For this review, take the finished solid that the model builds, in its own axes (mm). Give positions to 0.01 mm unless a question says otherwise; leave off trailing zeros. Write each loop counter-clockwise with the first axis right and the second up, starting at its lowest first coordinate (ties: lowest second). Pieces come first, ordered by that corner, then holes. Notation, with made-up numbers: M 2,74 L 59,74 A20 ccw 59,97 Z; hole C 51,24 d1. An arc over 180 degrees is marked long. Write item = value, one per line.
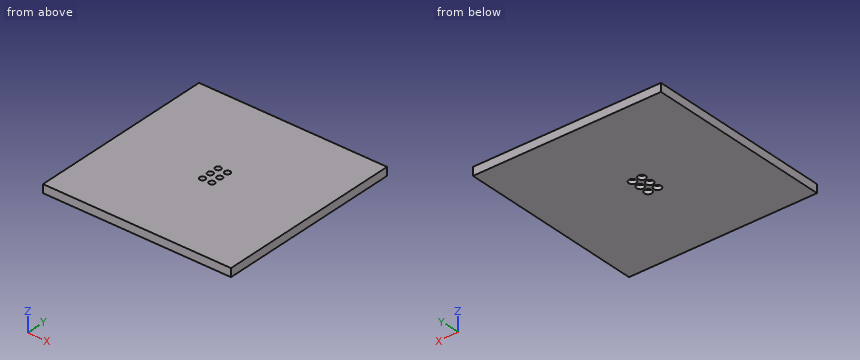
```python
from build123d import *

# Parameters (mm, degrees)
F0_W     = 50
F0_H     = 50
F0_R     = 0.75
F1_DEPTH = 1.2
F2_W     = 50
F2_H     = 50
F2_R     = 1
F3_DEPTH = 1


with BuildPart() as f1:
    # F0 (on Top) → F1 (new body)
    with BuildSketch(Plane.XY):
        Rectangle(F0_W, F0_H)
        with Locations((-1.25, -2.5)):
            Circle(F0_R, mode=Mode.SUBTRACT)
        with Locations((1.25, -2.5)):
            Circle(F0_R, mode=Mode.SUBTRACT)
        with Locations((-1.25, 0)):
            Circle(F0_R, mode=Mode.SUBTRACT)
        with Locations((-1.25, 2.5)):
            Circle(F0_R, mode=Mode.SUBTRACT)
        with Locations((1.25, 0)):
            Circle(F0_R, mode=Mode.SUBTRACT)
        with Locations((1.25, 2.5)):
            Circle(F0_R, mode=Mode.SUBTRACT)
    extrude(amount=F1_DEPTH)

    # F2 (on face) → F3 (join)
    with BuildSketch(Plane(origin=(0, 0, 0), x_dir=(1, 0, 0), z_dir=(0, 0, -1))):
        Rectangle(F2_W, F2_H)
        with Locations((-1.25, -2.5)):
            Circle(F2_R, mode=Mode.SUBTRACT)
        with Locations((1.25, -2.5)):
            Circle(F2_R, mode=Mode.SUBTRACT)
        with Locations((-1.25, 0)):
            Circle(F2_R, mode=Mode.SUBTRACT)
        with Locations((-1.25, 2.5)):
            Circle(F2_R, mode=Mode.SUBTRACT)
        with Locations((1.25, 0)):
            Circle(F2_R, mode=Mode.SUBTRACT)
        with Locations((1.25, 2.5)):
            Circle(F2_R, mode=Mode.SUBTRACT)
    extrude(amount=F3_DEPTH)


solid = f1.part
```
1. We need section B-B, the plane y = 2.5. Write out the cut boundary in (x, z), then the cut area to 3 significant figures.
Responses:
outline = M -25,-1 L -2.25,-1 L -2.25,0 L -2,0 L -2,1.2 L -25,1.2 Z; M -0.5,0 L -0.25,0 L -0.25,-1 L 0.25,-1 L 0.25,0 L 0.5,0 L 0.5,1.2 L -0.5,1.2 Z; M 2,0 L 2.25,0 L 2.25,-1 L 25,-1 L 25,1.2 L 2,1.2 Z
area = 102 mm2
2. For line 1 along Y through (x, z) = (-1.25, 0.75); line 2 along Y through (x, z) = (1.25, -0.55); line 3 along X through (y, z) = (0, -0.5), list the stretches that pass through material, from the lowest coordinate up. Write a range as from..to.
Responses:
line_1 = -25..-3.25, -1.75..-0.75, 0.75..1.75, 3.25..25
line_2 = -25..-3.5, -1.5..-1, 1..1.5, 3.5..25
line_3 = -25..-2.25, -0.25..0.25, 2.25..25
3. We need section A-A, the plane x = -1.25. Write out the cut boundary in (y, z).
Responses:
outline = M -25,-1 L -3.5,-1 L -3.5,0 L -3.25,0 L -3.25,1.2 L -25,1.2 Z; M -1.75,0 L -1.5,0 L -1.5,-1 L -1,-1 L -1,0 L -0.75,0 L -0.75,1.2 L -1.75,1.2 Z; M 0.75,0 L 1,0 L 1,-1 L 1.5,-1 L 1.5,0 L 1.75,0 L 1.75,1.2 L 0.75,1.2 Z; M 3.25,0 L 3.5,0 L 3.5,-1 L 25,-1 L 25,1.2 L 3.25,1.2 Z
4. Insertion check: P1, Ø1.7, axis at x = -1.25, y = -2.5, coming from the -Z side; P2, Ø2.5, axis at x = -1.25, y = 0, coming from the +Z side; P3, Ø1.4, axis at x = -1.25, y = 2.5, coming from the -Z side. Each pin has a flat end and moves straight along its axis. Give the tip position at first contact, or say it passes through.
Responses:
P1 = 0
P2 = 1.2
P3 = through
